Autodesk Inventor part; units mm, degrees
ref_plane "YZ Plane" through (0, 0, 0) normal (1, 0, 0) x (0, 1, 0)
ref_plane "XZ Plane" through (0, 0, 0) normal (0, 1, 0) x (-1, 0, 0)
ref_plane "XY Plane" through (0, 0, 0) normal (0, 0, 1) x (1, 0, 0)
ref_plane "Work Plane1" through (0, 0, 0) normal (0, 0, 1) x (1, 0, 0)
sketch "Sketch1" plane through (0, 0, 0) normal (0, 0, 1) x (1, 0, 0)
  line L0 (-44.1325, -41.275) -> (44.1325, -41.275)
  line L1 (44.1325, -41.275) -> (44.1325, 41.275)
  line L2 (44.1325, 41.275) -> (-44.1325, 41.275)
  line L3 (-44.1325, 41.275) -> (-44.1325, -41.275)
  line L4 (-44.1325, -41.275) -> (44.1325, 41.275) construction
  line L5 (44.1325, -41.275) -> (-44.1325, 41.275) construction
  line L6 (-45.4025, -42.545) -> (45.4025, -42.545)
  line L7 (45.4025, -42.545) -> (45.4025, 42.545)
  line L8 (45.4025, 42.545) -> (-45.4025, 42.545)
  line L9 (-45.4025, 42.545) -> (-45.4025, -42.545)
  line L10 (-45.4025, -42.545) -> (45.4025, 42.545) construction
  line L11 (45.4025, -42.545) -> (-45.4025, 42.545) construction
  point P0 (0, 0)
  dimension "d1" = 88.265
  dimension "d2" = 82.55
  dimension "d3" = 90.805
  dimension "d4" = 85.09
extrude "Extrusion1" add sketch "Sketch1" against normal blind 27.94
sketch "Sketch2" plane through (0, 0, 0) normal (0, 0, 1) x (1, 0, 0)
  line L0 (44.1325, 41.275) -> (-44.1325, 41.275)
  line L1 (-44.1325, -41.275) -> (44.1325, -41.275)
  line L2 (-44.1325, 41.275) -> (44.1325, 41.275)
  line L3 (44.1325, 41.275) -> (44.1325, -41.275)
  line L4 (44.1325, -41.275) -> (-44.1325, -41.275)
  line L5 (-44.1325, -41.275) -> (-44.1325, 41.275)
  point P0 (0, 0)
extrude "Extrusion2" add sketch "Sketch2" against normal blind 2.54
sketch "Sketch5" plane through (0, 0, 0) normal (0, 0, 1) x (1, 0, 0)
  line L0 (-45.4025, 42.545) -> (45.4025, 42.545)
  line L1 (-5.1231, 42.545) -> (4.8162, 42.545)
  line L2 (4.8162, 42.545) -> (4.8162, 17.0095)
  line L3 (4.8162, 17.0095) -> (-5.1231, 17.0095)
  line L4 (-5.1231, 17.0095) -> (-5.1231, 42.545)
  point P0 (0, 0)
extrude "Extrusion3" cut sketch "Sketch5" against normal up to next
sketch "Sketch6" plane through (0, 0, 0) normal (0, 0, 1) x (1, 0, 0)
  line L0 (-45.4025, 42.545) -> (-5.1231, 42.545)
  line L1 (-11.7648, 42.545) -> (10.5336, 42.545)
  line L2 (10.5336, 42.545) -> (10.5336, 5.472)
  line L3 (10.5336, 5.472) -> (-11.7648, 5.472)
  line L4 (-11.7648, 5.472) -> (-11.7648, 42.545)
  point P0 (0, 0)
extrude "Extrusion4" cut sketch "Sketch6" against normal up to next
sketch "Sketch7" plane through (0, 0, 0) normal (0, 0, 1) x (1, 0, 0)
  line L0 (13.9536, 42.6816) -> (-11.7648, 42.6816)
  line L1 (-11.7648, 42.6816) -> (-11.7648, 0)
  line L2 (-11.7648, 0) -> (13.9536, 0)
  line L3 (13.9536, 0) -> (13.9536, 42.6816)
  point P0 (0, 0)
extrude "Extrusion5" cut sketch "Sketch7" against normal up to next
sketch "Sketch8" plane through (0, 0, 0) normal (0, 0, 1) x (1, 0, 0)
  point P0 (0, 0)
Part model, mm, in its own coordinate system. A direction names the side the tool comes from. Coordinates: 2 decimals unless noted, no trailing zeros. Loops run counter-clockwise (first coordinate to the right, second up) from the corner with the lowest first, then second, coordinate; pieces in that order, holes last. Notation, with made-up numbers: (-18.75, 85.5) -> (28.25, 85.5) arc R16 ccw to (28.25, 112.5) -> close; hole circle Ø11 at (-4.5, 34). An arc over 180 degrees is marked (long way). Use a Markdown table: item, result. Add a question column.
Item 1: Band-saw the part on D-D on x = 7. Write the cut outline in (y, z) (3 decimals), plus the area to 3 significant figures.
Item 2: Band-saw the part on C-C on y = -27.5. Write the cut outline in (x, z).
Item 3: Band-saw the part on B-B on z = -18. Write the cut outline in (x, y) (1 decimal), plus the area to 3 significant figures.
Item 4: Band-saw the part on A-A on y = 24. Write the cut outline in (x, z), plus the area to 3 significant figures.
Item 5: Flat gauge pins, fed straight in: P1, Ø25, axis at x = 11.5, y = 4, coming from the -Z side; P2, Ø1.3, axis at x = 2, z = -1, coming from the +Y side. Where does each tip first touch, or does it go through?
Item 6: Pull direction Y, two halves, no side cores. Call faces 1 (the flat face through (44.132, -1, -15)), 2 (the flat face through (-1, -9, -2.54)), 3 (the flat face through (-28, 42.545, -14)), 4 (the flat face through (-1, -42.545, -14)): +Y half, -Y half, draft (parallel to the pull), parting line (faces both ways), or undercut.
Item 7: Which spindle directions (+Z, -Z, +X, -X, +Y, -Y) get a long thin tool onto all of the face, cutting with end or side? Do faces 5 (the flat face through (-44.132, 1, -15)), 6 (the flat face through (13.954, 26, -1)), 7 (the flat face through (45.402, -1, -14)). Say none if no direction does.
Item 8: Probe probe 1 along Y at (x, z) = (-33, -10.25) (3 decimals); probe 2 along X at (y, z) = (-35.5, -16.25); probe 3 along Y at (x, z) = (4.5, -18.25) (3 decimals). List the from-to ranges inside material, lowest first.
Geometry says:
| question | item | result |
|---|---|---|
| 1 | outline | (-42.545, -27.94) -> (-41.275, -27.94) -> (-41.275, -2.54) -> (0, -2.54) -> (0, 0) -> (-42.545, 0) -> close |
| 1 | area | 140 mm² |
| 2 | outline | (-45.4, -27.94) -> (-44.13, -27.94) -> (-44.13, -2.54) -> (44.13, -2.54) -> (44.13, -27.94) -> (45.4, -27.94) -> (45.4, 0) -> (-45.4, 0) -> close |
| 3 | outline | (-45.4, -42.5) -> (45.4, -42.5) -> (45.4, 42.5) -> (14, 42.5) -> (14, 41.3) -> (44.1, 41.3) -> (44.1, -41.3) -> (-44.1, -41.3) -> (-44.1, 41.3) -> (-11.8, 41.3) -> (-11.8, 42.5) -> (-45.4, 42.5) -> close |
| 3 | area | 408 mm² |
| 4 | outline | (-45.4, -27.94) -> (-44.13, -27.94) -> (-44.13, -2.54) -> (-11.76, -2.54) -> (-11.76, 0) -> (-45.4, 0) -> close; (13.95, -2.54) -> (44.13, -2.54) -> (44.13, -27.94) -> (45.4, -27.94) -> (45.4, 0) -> (13.95, 0) -> close |
| 4 | area | 230 mm² |
| 5 | P1 | z = -2.54 |
| 5 | P2 | y = 0 |
| 6 | face 1 | undercut |
| 6 | face 2 | undercut |
| 6 | face 3 | +Y half |
| 6 | face 4 | -Y half |
| 7 | face 5 | -Z |
| 7 | face 6 | +Z, -Z, +Y |
| 7 | face 7 | +Z, -Z, +X, +Y, -Y |
| 8 | probe 1 | -42.545 to -41.275, 41.275 to 42.545 |
| 8 | probe 2 | -45.4 to -44.13, 44.13 to 45.4 |
| 8 | probe 3 | -42.545 to -41.275 |
